from build123d import *

# Parameters (mm, degrees)
F0_W     = 25.4
F0_H     = 25.4
F1_DEPTH = 31.75
F2_R     = 11.43
F3_DEPTH = 12.7
F4_SIZE  = 2.54
F5_R     = 1.27
F6_R     = 1.26999
F7_R     = 11.43
F8_DEPTH = 12.7


# Not quite as in the source:
# - a fillet or chamfer is up to 0.001 mm smaller than in the source, because OpenCascade refuses the exact size


with BuildPart() as f1:
    # F0 (on Top) → F1 (new body)
    with BuildSketch(Plane.XY):
        Rectangle(F0_W, F0_H)
    extrude(amount=F1_DEPTH)

    # F2 (on face) → F3 (join)
    with BuildSketch(Plane.XY.offset(31.75)):
        Circle(F2_R)
    extrude(amount=F3_DEPTH)

    # F4
    f4_edges = [f1.edges().sort_by_distance(p)[0] for p in [
        (-11.43, 0, 44.45),
    ]]
    chamfer(f4_edges, length=F4_SIZE)

    # F5
    f5_edges = [f1.edges().sort_by_distance(p)[0] for p in [
        (-12.7, -12.7, 15.875),
        (12.7, -12.7, 15.875),
        (-12.7, 12.7, 15.875),
        (12.7, 12.7, 15.875),
    ]]
    fillet(f5_edges, radius=F5_R)

    # F6 (radius 1.27 in the source; OpenCascade refuses exactly that, so slightly less here)
    f6_edges = [f1.edges().sort_by_distance(p)[0] for p in [
        (0, -12.7, 31.75),
        (12.7, 0, 31.75),
        (0, 12.7, 31.75),
        (-12.7, 0, 31.75),
    ]]
    fillet(f6_edges, radius=F6_R)

    # F7 (on face) → F8 (cut)
    with BuildSketch(Plane(origin=(0, 0, 0), x_dir=(1, 0, 0), z_dir=(0, 0, -1))):
        Circle(F7_R)
    extrude(amount=-F8_DEPTH, mode=Mode.SUBTRACT)


solid = f1.part
Design review of the part built by this model. Coordinates are the model's own, in mm. A direction names the side the tool comes from. Round coordinates to 2 decimals unless told otherwise and drop trailing zeros. One line per item, written item: value. Start each with the question number.
1. To check wall thickness, follow probe 1 along X at (y, z) = (0, 9); probe 2 along Z at (x, y) = (-0.5, -2). State the ranges of each line that lie inside material, in increasing order. Write a range as from..to.
2. Draft analysis for pull direction X (two halves, no side actions). For faces 1 (the face through (12.318, 0.16, 31.388)), 2 (the face through (10.902, 3.433, 36.759)), 3 (the face through (0, 0, 12.7)), 4 (the face through (0, -12.7, 15)), state which applies: pulls with the +X half, pulls with the -X half, needs draft (parallel to the pull), parting line crosses it, or undercut.
3. For faces 5 (the face through (0, 12.7, 15)), 6 (the face through (10.902, -3.433, 6.261)), 7 (the face through (-8, 9, 31.75)), list the 3-axis set-ups (+Z, -Z, +X, -X, +Y, -Y) from which the entire face can be reached by the end or side of a thin tool; tool diameter is ignored.
4. Clearance check with flat-ended pins moving along their axes: P1, Ø5, axis at y = -5.5, z = 39, coming from the +X side; P2, Ø2, axis at y = -4.5, z = 39, coming from the +X side; P3, Ø1, axis at x = -6.5, y = 7, coming from the +Z side. State where each tip first meets the part, or that it passes through.
Computed:
1. probe 1: x = -12.7..-11.43, 11.43..12.7
1. probe 2: z = 12.7..44.45
2. face 1: pulls with the +X half
2. face 2: parting line crosses it
2. face 3: undercut
2. face 4: needs draft
3. face 5: +Z, -Z, +X, -X, +Y
3. face 6: -Z
3. face 7: +Z, +Y
4. P1: stops at x = 11.03
4. P2: stops at x = 10.88
4. P3: stops at z = 44.29
